from build123d import *

# Parameters (mm, degrees)
SKETCH1_R           = 1.5
SKETCH1_R_2         = 2
SKETCH1_R_3         = 10
BOSS_EXTRUDE1_DEPTH = 2


with BuildPart() as part:
    # Sketch1 → Boss-Extrude1 (new body)
    with BuildSketch(Plane.XY):
        with BuildLine():
            ThreePointArc((-19.25, 25), (0, 44.25), (19.25, 25))
            Line((19.25, 25), (19.25, -25))
            Line((19.25, -25), (-19.25, -25))
            Line((-19.25, -25), (-19.25, 25))
        make_face()
        with Locations((-12.990381057, 17.5)):
            Circle(SKETCH1_R, mode=Mode.SUBTRACT)
        with Locations((12.990381057, 17.5)):
            Circle(SKETCH1_R, mode=Mode.SUBTRACT)
        with Locations((10, -15)):
            Circle(SKETCH1_R_2, mode=Mode.SUBTRACT)
        with Locations((-10, -15)):
            Circle(SKETCH1_R_2, mode=Mode.SUBTRACT)
        with Locations((0, 40)):
            Circle(SKETCH1_R, mode=Mode.SUBTRACT)
        with Locations((0, 25)):
            Circle(SKETCH1_R_3, mode=Mode.SUBTRACT)
    extrude(amount=BOSS_EXTRUDE1_DEPTH)


solid = part.part
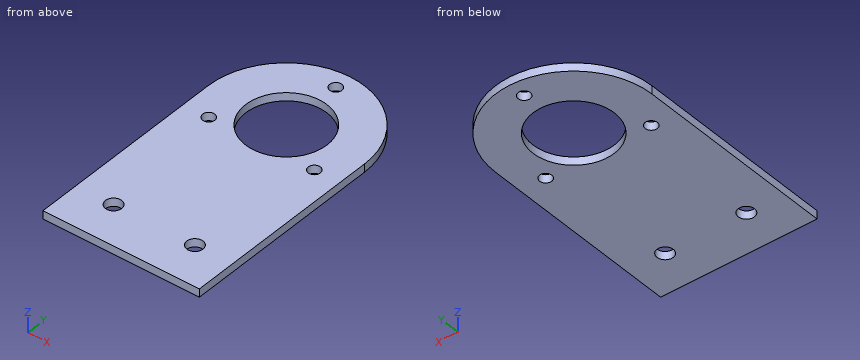
Can you work these out from the model? Positions are in its coordinate system, mm. Give positions to 0.01 mm unless a question says otherwise; leave off trailing zeros. Loops run counter-clockwise (first coordinate to the right, second up) from the corner with the lowest first, then second, coordinate; pieces in that order, holes last. Notation, with made-up numbers: (-8.5, -14.5) -> (18.5, -14.5) arc R20 ccw to (18.5, -1.5) -> close; hole circle Ø3 at (-22, 47). An arc over 180 degrees is marked (long way). Return JSON: item names as keys, results as strings.
Q1. I want a section at D-D, the plane x = 4. List the corners of the cut face in (y, z) for me.
Checks:
{"outline": "(-25, 0) -> (15.83, 0) -> (15.83, 2) -> (-25, 2) -> close; (34.17, 0) -> (43.83, 0) -> (43.83, 2) -> (34.17, 2) -> close"}
Q2. I want a section at B-B, the plane y = -15. List the corners of the cut face in (x, z) for me.
Checks:
{"outline": "(-19.25, 0) -> (-12, 0) -> (-12, 2) -> (-19.25, 2) -> close; (-8, 0) -> (8, 0) -> (8, 2) -> (-8, 2) -> close; (12, 0) -> (19.25, 0) -> (19.25, 2) -> (12, 2) -> close"}
Q3. I want a section at A-A, the plane x = 0. List the corners of the cut face in (y, z) for me, then the cut area to 3 significant figures.
Checks:
{"outline": "(-25, 0) -> (15, 0) -> (15, 2) -> (-25, 2) -> close; (35, 0) -> (38.5, 0) -> (38.5, 2) -> (35, 2) -> close; (41.5, 0) -> (44.25, 0) -> (44.25, 2) -> (41.5, 2) -> close", "area": "92.5 mm2"}
Q4. For pin 1 Ø16 at (x, y) = (0, 25) entering from -Z, with a flat end and sliding along its axis, tell me the tip position at first contact or that it passes through.
Checks:
{"pin 1": "passes through"}
Q5. I need wall thicknesses on probe 1 along Y at (x, z) = (1, 1.85); probe 2 along X at (y, z) = (27, 1.35); probe 3 along X at (y, z) = (32.5, 0.25). Which ranges of each line are inside material? Lowest first, please.
Checks:
{"probe 1": "y = -25 to 15.05, 34.95 to 38.88, 41.12 to 44.22", "probe 2": "x = -19.15 to -9.8, 9.8 to 19.15", "probe 3": "x = -17.73 to -6.61, 6.61 to 17.73"}
Q6. I want a section at C-C, the plane y = 17.5. List the corners of the cut face in (x, z) for me, then the cut area to 3 significant figures.
Checks:
{"outline": "(-19.25, 0) -> (-14.49, 0) -> (-14.49, 2) -> (-19.25, 2) -> close; (-11.49, 0) -> (-6.61, 0) -> (-6.61, 2) -> (-11.49, 2) -> close; (6.61, 0) -> (11.49, 0) -> (11.49, 2) -> (6.61, 2) -> close; (14.49, 0) -> (19.25, 0) -> (19.25, 2) -> (14.49, 2) -> close", "area": "38.5 mm2"}
